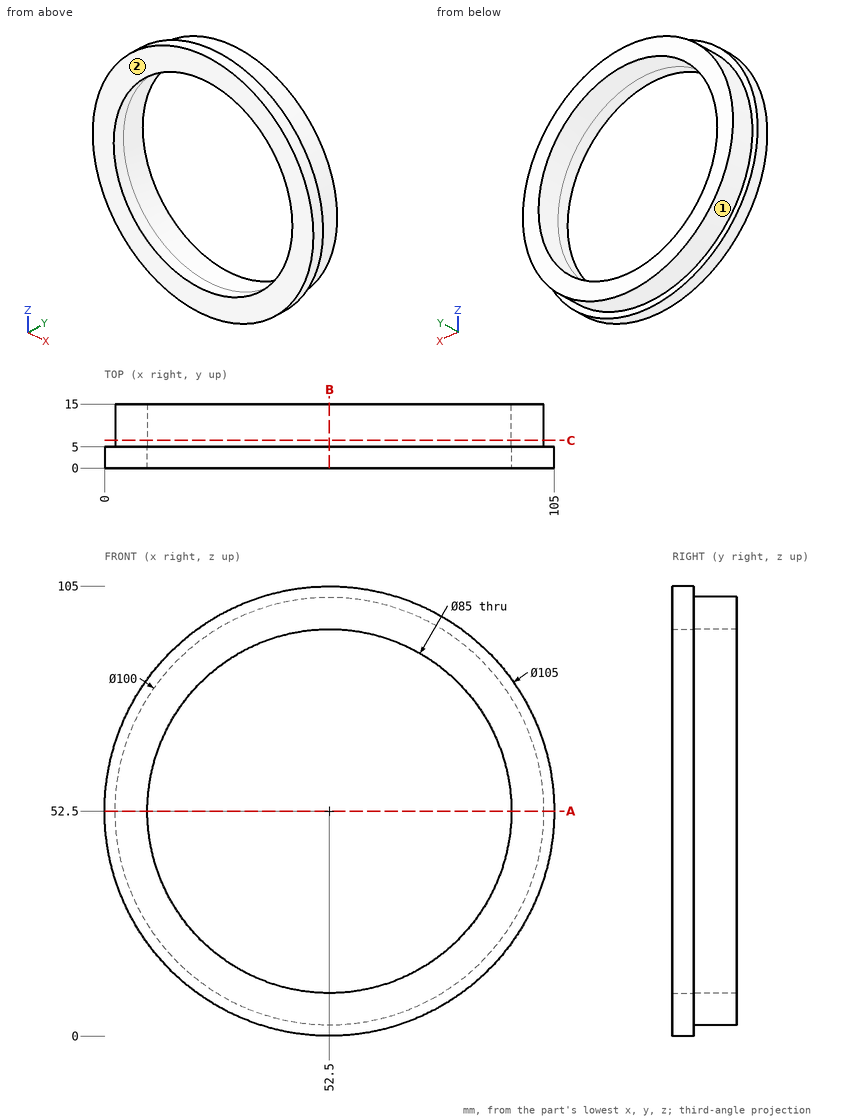
The figure shows three views and two pictorial views of one solid part (mm, origin at its lowest corner). Answer the questions. A direction names the side the tool comes from. Round coordinates to 2 decimals unless told otherwise and drop trailing zeros. Loops run counter-clockwise (first coordinate to the right, second up) from the corner with the lowest first, then second, coordinate; pieces in that order, holes last. Notation, with made-up numbers: M 88,-27 L 99,-27 A21 cw 99,10 Z; hole C 58,-12 d9. An arc over 180 degrees is marked long. Write each question's results on one line, items separated by ' | '. Start each with the question number.
1) Find section B-B on x = 52.5. Write down the section's boundary in (y, z), plus the area to 3 significant figures.
2) Find section C-C on y = 6.5. Write down the section's boundary in (x, z), plus the area to 3 significant figures.
3) Straight lines are drawn through the part: probe 1 along Z at (x, y) = (52.5, 3.3); probe 2 along X at (y, z) = (10.5, 52.5). For each, find the intervals that lie inside material, in ascending order.
4) Each of these flat-tipped pins is pushed along its axis until it touches: pin 1 (1 mm diameter, centred on y = 2, z = 71.5, fed in from -X); pin 2 (5 mm diameter, centred on y = 4, z = 18, fed in from +X); pin 3 (1.5 mm diameter, centred on x = 83, y = 7.5, fed in from +Z). Where does it stop, or does it pass through?
5) Find section A-A on z = 52.5. Write down the section's boundary in (x, y).
6) Which of the six approach directions +Z, -Z, +X, -X, +Y, -Y give full straight-line access (tool end or side, diameter ignored) to the marked faces 1 and 2?
Final values:
1) outline: M 0,0 L 5,0 L 5,2.5 L 15,2.5 L 15,10 L 0,10 Z; M 0,95 L 15,95 L 15,102.5 L 5,102.5 L 5,105 L 0,105 Z | area: 250 mm²
2) outline: C 52.5,52.5 d100; hole C 52.5,52.5 d85 | area: 2,180 mm²
3) probe 1: 0 to 10, 95 to 105 | probe 2: 2.5 to 10, 95 to 102.5
4) pin 1: x = 3.37 | pin 2: x = 94.12 | pin 3: z = 92.69
5) outline: M 0,0 L 10,0 L 10,15 L 2.5,15 L 2.5,5 L 0,5 Z; M 95,0 L 105,0 L 105,5 L 102.5,5 L 102.5,15 L 95,15 Z
6) face 1: +Y | face 2: +Z, -Z, +X, -X, -Y
